from build123d import *

# Parameters (mm, degrees)
BOSS_EXTRUDE1_DEPTH = 1.524


with BuildPart() as part:
    # Sketch1 → Boss-Extrude1 (new body)
    with BuildSketch(Plane.XY):
        with BuildLine():
            Line((0, -185.062075144), (-1.524, -185.062075144))
            Line((-1.524, -185.062075144), (-1.524, -147.624689716))
            ThreePointArc((-1.524, -147.624689716), (-6.010146882, -153.015597415), (-11.384626883, -157.521411923))
            Line((-11.384626883, -157.521411923), (-8.18166696, -177.565293098))
            Line((-8.18166696, -177.565293098), (-9.686574021, -177.80577332))
            Line((-9.686574021, -177.80577332), (-6.680571239, -196.617111584))
            Line((-6.680571239, -196.617111584), (-5.175664178, -196.376631362))
            Line((-5.175664178, -196.376631362), (-1.585117021, -218.846004156))
            Line((-1.585117021, -218.846004156), (0.061117021, -218.846004156))
            Line((0.061117021, -218.846004156), (3.651664178, -196.376631362))
            Line((3.651664178, -196.376631362), (5.156571239, -196.617111584))
            Line((5.156571239, -196.617111584), (8.162574021, -177.80577332))
            Line((8.162574021, -177.80577332), (6.65766696, -177.565293098))
            Line((6.65766696, -177.565293098), (9.860626883, -157.521411923))
            ThreePointArc((9.860626883, -157.521411923), (4.486146882, -153.015597415), (0, -147.624689716))
            Line((0, -147.624689716), (0, -185.062075144))
        make_face()
    extrude(amount=BOSS_EXTRUDE1_DEPTH)


solid = part.part
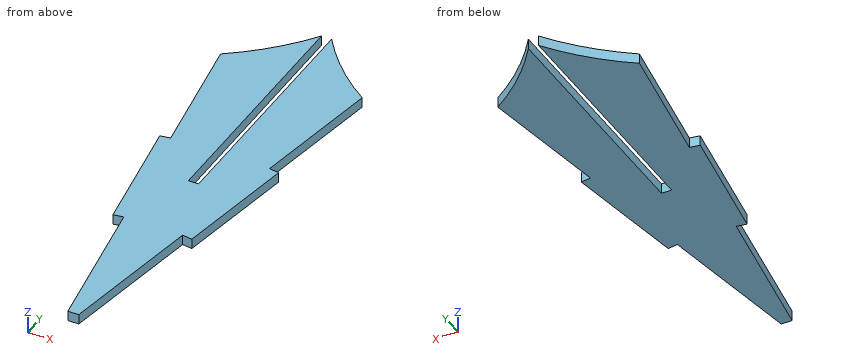
Work out the finished part from the listing and answer in its coordinate system (mm). Give positions to 0.01 mm unless a question says otherwise; leave off trailing zeros. Loops run counter-clockwise (first coordinate to the right, second up) from the corner with the lowest first, then second, coordinate; pieces in that order, holes last. Notation, with made-up numbers: (62.25, -24.75) -> (76.25, -24.75) arc R30 ccw to (76.25, 8.25) -> close; hole circle Ø2 at (52.5, 71.25). An arc over 180 degrees is marked (long way). Use a Markdown table: item, result. Add a question column.
1. Find the intervals of material crossed by probe 1 along X at (y, z) = (-167, 0.1); probe 2 along X at (y, z) = (-188.5, 0.5); probe 3 along X at (y, z) = (-201, 0.45), in increasing order.
2. Section C-C on y = -179.5 is taken. Determine the outline of the cut face in (x, z), and give its area (3 significant figures).
3. Section A-A on x = 7.5 is taken. Determine the outline of the cut face in (y, z).
4. Flat-ended cylindrical pins translate along their axes: pin 1 Ø10 at (x, y) = (6.5, -166.5) entering from -Z; pin 2 Ø0.5 at (y, z) = (-161.5, 0.5) entering from -X; pin 3 Ø0.5 at (y, z) = (-164, 1) entering from +X. Find the tip coordinate at first contact, or state that the pin passes through.
5. Section B-B on z = 0.95 is taken. Determine the outline of the cut face in (x, y).
6. Section D-D on y = -207 is taken. Determine the outline of the cut face in (x, z), and give its area (3 significant figures).
Results below:
| question | item | result |
|---|---|---|
| 1 | probe 1 | x = -9.87 to -1.52, 0 to 8.35 |
| 1 | probe 2 | x = -7.98 to 6.45 |
| 1 | probe 3 | x = -4.44 to 2.91 |
| 2 | outline | (-9.42, 0) -> (-1.52, 0) -> (-1.52, 1.52) -> (-9.42, 1.52) -> close; (0, 0) -> (7.89, 0) -> (7.89, 1.52) -> (0, 1.52) -> close |
| 2 | area | 24.1 mm^2 |
| 3 | outline | (-181.95, 0) -> (-177.7, 0) -> (-177.7, 1.52) -> (-181.95, 1.52) -> close; (-172.29, 0) -> (-155.74, 0) -> (-155.74, 1.52) -> (-172.29, 1.52) -> close |
| 4 | pin 1 | stops at z = 0 |
| 4 | pin 2 | stops at x = -10.79 |
| 4 | pin 3 | stops at x = 8.87 |
| 5 | outline | (-11.38, -157.52) -> (-8.18, -177.57) -> (-9.69, -177.81) -> (-6.68, -196.62) -> (-5.18, -196.38) -> (-1.59, -218.85) -> (0.06, -218.85) -> (3.65, -196.38) -> (5.16, -196.62) -> (8.16, -177.81) -> (6.66, -177.57) -> (9.86, -157.52) arc R39.22 cw to (0, -147.62) -> (0, -185.06) -> (-1.52, -185.06) -> (-1.52, -147.62) arc R39.22 cw to start |
| 6 | outline | (-3.48, 0) -> (1.95, 0) -> (1.95, 1.52) -> (-3.48, 1.52) -> close |
| 6 | area | 8.28 mm^2 |
